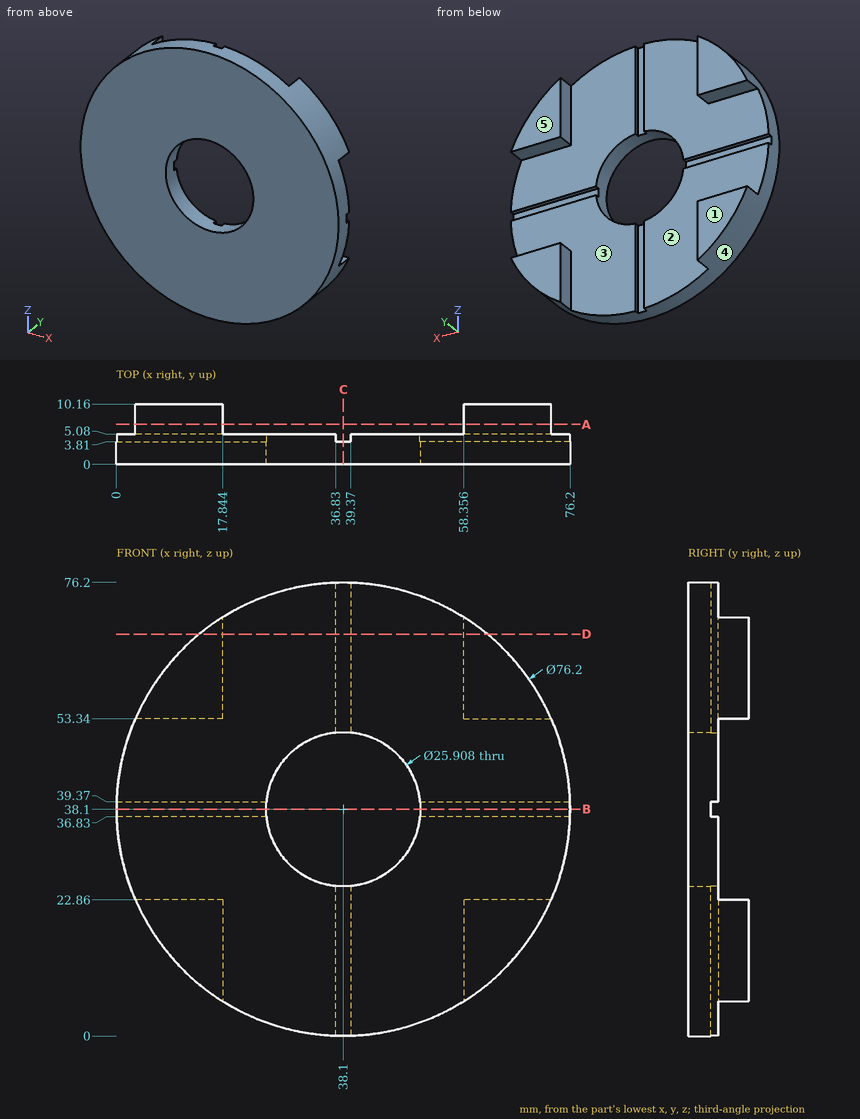
The drawing under review shows one solid part. Ordinate dimensions are in mm from its lowest x, y, z. A direction names the side the tool comes from. Give positions to 0.01 mm unless a question says otherwise; leave off trailing zeros. Order: outer loops, then holes, each group sorted by start corner. A loop starts at its lowest first (then second) coordinate and runs counter-clockwise, first axis right, second up. Notation, with made-up numbers: M -0.5,23 L 12.5,23 A34 ccw 12.5,56 Z; hole C 36.5,22 d10. An arc over 180 degrees is marked long. Answer in a Markdown table with one row per item. Add a question column.
1. Machinability: for the marked faces 1 and 2, which of the approach directions +Z, -Z, +X, -X, +Y, -Y give a long, thin tool a straight path to every point of the face, cutting with its end or side? Answer none if there is none.
2. For pin 1 Ø5.5 at (x, y) = (68.5, 8) entering from +Z; pin 2 Ø1.5 at (x, y) = (9.5, 8.5) entering from +Z; pin 3 Ø11 at (x, z) = (50.5, 18.5) entering from +Y, all flat-tipped, find the tip position at first contact; note any pin that passes through.
3. Mouldability with a two-part tool opening along X and no side actions: class the marked faces 3, 4 and 5 as released by +X, released by -X, zero draft, split by the parting line, or undercut.
4. Add section C-C on x = 38.1. State the section outline as (y, z) points (1 decimal).
5. Add section A-A on y = 6.75. State the section outline as (x, z) points.
6. Add section D-D on z = 67.5. State the section outline as (x, y) points.
7. To check wall thickness, follow line 1 along Z through (x, y) = (39.5, 4.25) (1 decimal); line 2 along Z through (x, y) = (38.1, 1.7) (1 decimal). State the ranges of each line that lie inside material, in increasing order.
8. Add section B-B on z = 38.1. State the section outline as (x, y) points (1 decimal).
The answers:
| question | item | result |
|---|---|---|
| 1 | face 1 | +Z, -Z, +X, -X, +Y |
| 1 | face 2 | +Y |
| 2 | pin 1 | z = 64.31 |
| 2 | pin 2 | z = 64.1 |
| 2 | pin 3 | y = 5.08 |
| 3 | face 3 | undercut |
| 3 | face 4 | split by the parting line |
| 3 | face 5 | zero draft |
| 4 | outline | M 0,0 L 3.8,0 L 3.8,25.1 L 0,25.1 Z; M 0,51.1 L 3.8,51.1 L 3.8,76.2 L 0,76.2 Z |
| 5 | outline | M 3.18,22.86 A38.1 ccw 17.84,5.83 L 17.84,22.86 Z; M 3.18,53.34 L 17.84,53.34 L 17.84,70.37 A38.1 ccw Z; M 58.36,5.83 A38.1 ccw 73.02,22.86 L 58.36,22.86 Z; M 58.36,53.34 L 73.02,53.34 A38.1 ccw 58.36,70.37 Z |
| 6 | outline | M 13.87,0 L 62.33,0 L 62.33,10.16 L 58.36,10.16 L 58.36,5.08 L 39.37,5.08 L 39.37,3.81 L 36.83,3.81 L 36.83,5.08 L 17.84,5.08 L 17.84,10.16 L 13.87,10.16 Z |
| 7 | line 1 | 0 to 25.2, 51 to 76.2 |
| 7 | line 2 | 0 to 25.1, 51.1 to 76.2 |
| 8 | outline | M 0,0 L 25.1,0 L 25.1,3.8 L 0,3.8 Z; M 51.1,0 L 76.2,0 L 76.2,3.8 L 51.1,3.8 Z |
